Input: part model. Units: mm. Frame: model coordinates. Give positions to 0.01 mm unless a question says otherwise; leave off trailing zeros. Write each loop counter-clockwise with the first axis right and the second up, starting at its lowest first coordinate (ties: lowest second). Pieces come first, ordered by that corner, then holes.
```python
from build123d import *

# Parameters (mm, degrees)
BOSS_EXTRUDE1_DEPTH = 3.175
SKETCH2_R           = 2.05
CUT_EXTRUDE1_DEPTH  = 4.175
SKETCH3_W           = 3.175
SKETCH3_H           = 15
BOSS_EXTRUDE2_DEPTH = 3.175
FILLET1_R           = 1


with BuildPart() as part:
    # Sketch1 → Boss-Extrude1 (new body)
    with BuildSketch(Plane.XY):
        Polygon((-31.75, -60), (-15, -60), (-15, -63.175), (15, -63.175), (15, -60), (31.75, -60), (43.75, -60), (43.75, -53), (31.75, -14.842431943), (31.75, 60), (-31.75, 60), (-31.75, -14.842431943), (-43.75, -14.842431943), (-43.75, -53), (-43.75, -60), align=None)
    extrude(amount=BOSS_EXTRUDE1_DEPTH)

    # Sketch2 → Cut-Extrude1 (cut, through all)
    with BuildSketch(Plane.XY.offset(3.175)):
        with Locations((23.75, 30)):
            Circle(SKETCH2_R)
        with Locations((23.75, -40)):
            Circle(SKETCH2_R)
        with Locations((-23.75, -40)):
            Circle(SKETCH2_R)
        with Locations((-23.75, 30)):
            Circle(SKETCH2_R)
    extrude(amount=-CUT_EXTRUDE1_DEPTH, mode=Mode.SUBTRACT)

    # Sketch3 → Boss-Extrude2 (add)
    with BuildSketch(Plane.ZY.offset(43.75)):
        with Locations((1.5875, -35.5)):
            Rectangle(SKETCH3_W, SKETCH3_H)
    extrude(amount=BOSS_EXTRUDE2_DEPTH)

    # Fillet1
    fillet1_edges = [part.edges().sort_by_distance(p)[0] for p in [
        (15, -63.175, 1.5875),
        (-15, -63.175, 1.5875),
        (-46.925, -43, 1.5875),
        (-46.925, -28, 1.5875),
    ]]
    fillet(fillet1_edges, radius=FILLET1_R)


solid = part.part
```
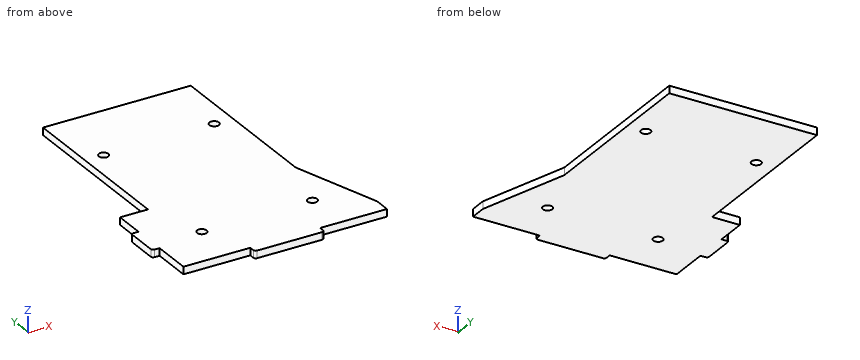
Q1. Section A-A, the plane y = 30. Return the cut outline in (x, z) (3 decimals).
Q2. Material intervals for line 1 along Y through (x, z) = (23.5, 1.7); line 2 along X through (y, z) = (-41, 1.45) (3 decimals); line 3 along X through (y, z) = (3, 1.25), sorted ascending.
Q3. Section D-D, the plane y = -45. Return the cut outline in (x, z) (3 decimals), then the cut area to 3 significant figures.
Q4. Section B-B, the plane z = 0.6. Return the cut outline in (x, y) (3 decimals).
Q5. Section C-C, the plane x = -23.75. Return the cut outline in (y, z) (3 decimals).
Q6. Pin query (flat end, axial travel): pin 1 (1.5 mm diameter, centred on y = -17, z = 0.5, fed in from -X); pin 2 (6 mm diameter, centred on x = 4.5, y = 8, fed in from -Z); pin 3 (1.6 mm diameter, centred on x = -29.5, z = 2.5, fed in from -Y); pin 4 (1.7 mm diameter, centred on x = -45, z = 1.5, fed in from -Y). Return the tip coordinate at first contact, or that it passes through.
Solutions:
1. outline: (-31.75, 0) - (-25.8, 0) - (-25.8, 3.175) - (-31.75, 3.175) - close; (-21.7, 0) - (21.7, 0) - (21.7, 3.175) - (-21.7, 3.175) - close; (25.8, 0) - (31.75, 0) - (31.75, 3.175) - (25.8, 3.175) - close
2. line 1: y = -60 to -42.03, -37.97 to 27.97, 32.03 to 60
2. line 2: x = -46.925 to -25.54, -21.96 to 21.96, 25.54 to 39.976
2. line 3: x = -31.75 to 31.75
3. outline: (-43.75, 0) - (41.234, 0) - (41.234, 3.175) - (-43.75, 3.175) - close
3. area: 270 mm2
4. outline: (-46.925, -42) arc R1 ccw to (-45.925, -43) - (-43.75, -43) - (-43.75, -60) - (-15, -60) - (-15, -62.175) arc R1 ccw to (-14, -63.175) - (14, -63.175) arc R1 ccw to (15, -62.175) - (15, -60) - (43.75, -60) - (43.75, -53) - (31.75, -14.842) - (31.75, 60) - (-31.75, 60) - (-31.75, -14.842) - (-43.75, -14.842) - (-43.75, -28) - (-45.925, -28) arc R1 ccw to (-46.925, -29) - close; hole circle Ø4.1 at (-23.75, -40); hole circle Ø4.1 at (-23.75, 30); hole circle Ø4.1 at (23.75, -40); hole circle Ø4.1 at (23.75, 30)
5. outline: (-60, 0) - (-42.05, 0) - (-42.05, 3.175) - (-60, 3.175) - close; (-37.95, 0) - (27.95, 0) - (27.95, 3.175) - (-37.95, 3.175) - close; (32.05, 0) - (60, 0) - (60, 3.175) - (32.05, 3.175) - close
6. pin 1: stops at x = -43.75
6. pin 2: stops at z = 0
6. pin 3: stops at y = -60
6. pin 4: stops at y = -43
